```python
from build123d import *

# Parameters (mm, degrees)
SKETCH1_W                       = 0.5
SKETCH1_H                       = 16
SKETCH1_H_2                     = 1
SKETCH1_H_3                     = 3
BOSS_EXTRUDE1_DEPTH             = 15
SKETCH5_W                       = 2
SKETCH5_H                       = 3
CUT_EXTRUDE1_DEPTH              = 2
BOSS_EXTRUDE2_DEPTH             = 2
STICK_START                     = -2.8
STICK_OUTS_DEPTH                = 0.8
PIN_HOLE_SKETCH_R               = 2
PIN_HOLE_DEPTH                  = 5.183346
PIN_HOLE_DIRECTION_2_REACH      = 29.406
PIN_HOLE_DIRECTION_2_END_RADIUS = 11


with BuildPart() as part:
    # Sketch1 → Boss-Extrude1 (new body)
    with BuildSketch(Plane.XY):
        with BuildLine():
            Line((-2, -5.183346174), (-2, 10.816653826))
            ThreePointArc((-2, 10.816653826), (-7.03562364, -8.455767263), (11, 0))
            ThreePointArc((11, 0), (8.455767263, 7.03562364), (2, 10.816653826))
            Line((2, 10.816653826), (2, -5.183346174))
            Line((2, -5.183346174), (2, -6.183346174))
            Line((2, -6.183346174), (2, -9.183346174))
            Line((2, -9.183346174), (1.5, -9.183346174))
            Line((1.5, -9.183346174), (-1.5, -9.183346174))
            Line((-1.5, -9.183346174), (-2, -9.183346174))
            Line((-2, -9.183346174), (-2, -6.183346174))
            Line((-2, -6.183346174), (-1.5, -6.183346174))
            Line((-1.5, -6.183346174), (-1, -6.183346174))
            Line((-1, -6.183346174), (-1, -5.183346174))
            Line((-1, -5.183346174), (-1.5, -5.183346174))
            Line((-1.5, -5.183346174), (-2, -5.183346174))
        make_face()
        with Locations((1.75, 2.816653826)):
            Rectangle(SKETCH1_W, SKETCH1_H)
        with Locations((1.75, -5.683346174)):
            Rectangle(SKETCH1_W, SKETCH1_H_2)
        with Locations((1.75, -7.683346174)):
            Rectangle(SKETCH1_W, SKETCH1_H_3)
        with Locations((-1.75, -7.683346174)):
            Rectangle(SKETCH1_W, SKETCH1_H_3)
        with Locations((-1.75, 2.816653826)):
            Rectangle(SKETCH1_W, SKETCH1_H)
        with BuildLine():
            ThreePointArc((2, 10.816653826), (1.75046389, 10.859828552), (1.5, 10.897247359))
            Line((1.5, 10.897247359), (1.5, 10.816653826))
            Line((1.5, 10.816653826), (2, 10.816653826))
        make_face()
        with BuildLine():
            Line((-1.5, 10.816653826), (-1.5, 10.897247359))
            ThreePointArc((-1.5, 10.897247359), (-1.75046389, 10.859828552), (-2, 10.816653826))
            Line((-2, 10.816653826), (-1.5, 10.816653826))
        make_face()
    extrude(amount=BOSS_EXTRUDE1_DEPTH)

    # Sketch5 → Cut-Extrude1 (cut)
    with BuildSketch(Plane(origin=(0, 0, 0), x_dir=(-1, 0, 0), z_dir=(0, 0, -1))):
        with Locations((-5, 0)):
            Rectangle(SKETCH5_W, SKETCH5_H)
        with Locations((5, 0)):
            Rectangle(SKETCH5_W, SKETCH5_H)
    extrude(amount=-CUT_EXTRUDE1_DEPTH, mode=Mode.SUBTRACT)

    # Sketch3 → Boss-Extrude2 (add)
    with BuildSketch(Plane.XY.offset(15)):
        with BuildLine():
            add(Edge.make_bspline(
                [(-14.354093493, -5), (-12.863344749, -9.279669369), (-8.266658173, -12.812493902), (-2.2, -12.812493902)],
                knots=[0, 0, 0, 0, 1, 1, 1, 1], degree=3))
            ThreePointArc((-2.2, -12.812493902), (-8.103626672, -10.165197232), (-12, -5))
            Line((-12, -5), (-14.354093493, -5))
        make_face()
        with BuildLine():
            Line((-2.2, -12.812493902), (2.2, -12.812493902))
            ThreePointArc((2.2, -12.812493902), (8.103626672, -10.165197232), (12, -5))
            Line((12, -5), (9.797958971, -5))
            ThreePointArc((9.797958971, -5), (0, -11), (-9.797958971, -5))
            Line((-9.797958971, -5), (-12, -5))
            ThreePointArc((-12, -5), (-8.103626672, -10.165197232), (-2.2, -12.812493902))
        make_face()
        with BuildLine():
            ThreePointArc((12, -5), (8.103626672, -10.165197232), (2.2, -12.812493902))
            add(Edge.make_bspline(
                [(2.2, -12.812493902), (6.731876181, -12.812493902), (12.505086924, -10.308162631), (14.354093493, -5)],
                knots=[0, 0, 0, 0, 1, 1, 1, 1], degree=3))
            Line((14.354093493, -5), (12, -5))
        make_face()
        with BuildLine():
            ThreePointArc((-9.797958971, -5), (0, -11), (9.797958971, -5))
            Line((9.797958971, -5), (1.5, -5))
            Line((1.5, -5), (1.5, -9.183346174))
            Line((1.5, -9.183346174), (-1.5, -9.183346174))
            Line((-1.5, -9.183346174), (-1.5, -6.183346174))
            Line((-1.5, -6.183346174), (-1, -6.183346174))
            Line((-1, -6.183346174), (-1, -5.183346174))
            Line((-1, -5.183346174), (-1.5, -5.183346174))
            Line((-1.5, -5.183346174), (-1.5, -5))
            Line((-1.5, -5), (-9.797958971, -5))
        make_face()
        with BuildLine():
            Line((1.5, -5), (9.797958971, -5))
            ThreePointArc((9.797958971, -5), (10.695268783, -2.571230378), (11, 0))
            ThreePointArc((11, 0), (8.291561976, 7.228416147), (1.5, 10.897247359))
            Line((1.5, 10.897247359), (1.5, -5))
        make_face()
        with BuildLine():
            ThreePointArc((-1.5, 10.897247359), (-9.751491559, 5.090030685), (-9.797958971, -5))
            Line((-9.797958971, -5), (-1.5, -5))
            Line((-1.5, -5), (-1.5, 10.897247359))
        make_face()
        with BuildLine():
            Line((9.797958971, -5), (12, -5))
            ThreePointArc((12, -5), (12.747548784, -2.549509757), (13, 0))
            ThreePointArc((13, 0), (-2.549509757, 12.747548784), (-12, -5))
            Line((-12, -5), (-9.797958971, -5))
            ThreePointArc((-9.797958971, -5), (-9.751491559, 5.090030685), (-1.5, 10.897247359))
            ThreePointArc((-1.5, 10.897247359), (0, 11), (1.5, 10.897247359))
            ThreePointArc((1.5, 10.897247359), (8.291561976, 7.228416147), (11, 0))
            ThreePointArc((11, 0), (10.695268783, -2.571230378), (9.797958971, -5))
        make_face()
        with BuildLine():
            ThreePointArc((13, 0), (12.747548784, -2.549509757), (12, -5))
            Line((12, -5), (14.354093493, -5))
            ThreePointArc((14.354093493, -5), (14.987031412, -2.535525479), (15.2, 0))
            ThreePointArc((15.2, 0), (-2.535525479, 14.987031412), (-14.354093493, -5))
            Line((-14.354093493, -5), (-12, -5))
            ThreePointArc((-12, -5), (-2.549509757, 12.747548784), (13, 0))
        make_face()
        with BuildLine():
            ThreePointArc((1.5, 10.897247359), (0, 11), (-1.5, 10.897247359))
            Line((-1.5, 10.897247359), (1.5, 10.897247359))
        make_face()
    extrude(amount=BOSS_EXTRUDE2_DEPTH)

    # Sketch6 → Stick Outs (add)
    with BuildSketch(Plane.XY.offset(17).offset(STICK_START)):
        with BuildLine():
            Line((-11.719212261, -2.066413314), (-10.832885283, -1.910129954))
            ThreePointArc((-10.832885283, -1.910129954), (-10.973204553, -0.767321211), (-10.993299097, 0.383894464))
            Line((-10.993299097, 0.383894464), (-11.892750842, 0.415304011))
            ThreePointArc((-11.892750842, 0.415304011), (-11.871012198, -0.830102038), (-11.719212261, -2.066413314))
        make_face()
    stick_outs = extrude(amount=STICK_OUTS_DEPTH)

    # Mirror1: Stick Outs across plane
    add(stick_outs.mirror(Plane(origin=(0, 0, 0), x_dir=(0, 0, 1), z_dir=(1, 0, 0))))

    # Pin Hole sketch → Pin hole (cut)
    with BuildSketch(Plane(origin=(0, 0, 0), x_dir=(1, 0, 0), z_dir=(0, 1, 0))):
        with Locations((0, -2)):
            Circle(PIN_HOLE_SKETCH_R)
    extrude(amount=-PIN_HOLE_DEPTH, mode=Mode.SUBTRACT)

    # Pin hole direction 2: up to this cylinder (the profile starts inside it)
    pin_hole_direction_2_end = Plane(origin=(0, 0, 2), z_dir=(0, 0, -1)) * Cylinder(PIN_HOLE_DIRECTION_2_END_RADIUS, 81.812, mode=Mode.PRIVATE)
    # Pin Hole sketch → Pin hole direction 2 (cut, up to the surface)
    with BuildSketch(Plane(origin=(0, 0, 0), x_dir=(1, 0, 0), z_dir=(0, 1, 0)), mode=Mode.PRIVATE) as pin_hole_direction_2_sk1:
        with Locations((0, -2)):
            Circle(PIN_HOLE_SKETCH_R)
    pin_hole_direction_2_tool1 = extrude(pin_hole_direction_2_sk1.sketch, amount=PIN_HOLE_DIRECTION_2_REACH, mode=Mode.PRIVATE) & pin_hole_direction_2_end
    add(pin_hole_direction_2_tool1.solids().sort_by_distance((0, 0, 2))[0], mode=Mode.SUBTRACT)


solid = part.part
```
Read the model definition and answer for the solid it produces. Units are mm, in the model's axes. A direction names the side the tool comes from. Round coordinates to 2 decimals unless told otherwise and drop trailing zeros. Write each loop counter-clockwise with the first axis right and the second up, starting at its lowest first coordinate (ties: lowest second). Pieces come first, ordered by that corner, then holes. Notation, with made-up numbers: (17, 87.5) -> (73, 87.5) arc R28 cw to (73, 113.5) -> close; hole circle Ø5 at (-9.5, -21). An arc over 180 degrees is marked (long way). Answer in a Markdown table with one row per item. Add a question column.
1) Find section D-D, the plane z = 1.5. Determine the outline of the cut face in (x, y).
2) Consider line 1 (X direction, y = 4.5, z = 4.75); line 2 (X direction, y = 5.75, z = 8.75); line 3 (Z direction, x = 12, y = -2.75). Determine where each line is inside the solid, lowest interval first.
3) Find section B-B, the plane y = 10. Determine the outline of the cut face in (x, z), and give its area (3 significant figures).
4) Find section A-A, the plane x = 0. Determine the outline of the cut face in (y, z), and give its area (3 significant figures).
5) Find section C-C, the plane z = 11. Determine the outline of the cut face in (x, y).
6) Given P1, Ø0.6, axis at x = -5.5, y = 0.5, coming from the -Z side; P2, Ø1.6, axis at x = -4.5, z = 0.5, coming from the -Y side; P3, Ø5, axis at x = 11, z = 9, coming from the +Y side, each flat-ended and moving along its own axis, determine where each tip first touches the part or whether it passes through.
7) Which of the six approach directions +Z, -Z, +X, -X, +Y, -Y give full straight-line access (tool end or side, diameter ignored) to faces 5 (the face through (11.28, -1.99, 14.59)), 6 (the face through (0, 10.897, 16)), 7 (the face through (5, 0, 2))?
8) Determine the mould class of faces 1 (the face through (4, 0, 1)), 2 (the face through (0, -12.812, 16)), 3 (the face through (11.872, -0.813, 14.594)), 4 (the face through (2, 3, 2)) for opening direction X: pulls with the +X half, pulls with the -X half, needs draft (parallel to the pull), parting line crosses it, or undercut.
Findings below:
| question | item | result |
|---|---|---|
| 1 | outline | (-2, 10.82) arc R11 ccw (long way) to (2, 10.82) arc R11 ccw to (1.94, 10.83) -> (1.94, -5.18) -> (1.5, -5.18) -> (1.5, -9.18) -> (-1.5, -9.18) -> (-1.5, -6.18) -> (-1, -6.18) -> (-1, -5.18) -> (-1.94, -5.18) -> (-1.94, 10.83) arc R11 ccw to start; hole (-6, -1.5) -> (-4, -1.5) -> (-4, 1.5) -> (-6, 1.5) -> close; hole (4, -1.5) -> (6, -1.5) -> (6, 1.5) -> (4, 1.5) -> close |
| 2 | line 1 | -10.04 to -1.5, 1.5 to 10.04 |
| 2 | line 2 | -9.38 to -1.5, 1.5 to 9.38 |
| 2 | line 3 | 15 to 17 |
| 3 | outline | (-11.45, 15) -> (-4.58, 15) -> (-4.58, 0) -> (-1.5, 0) -> (-1.5, 0.68) arc R2 cw to (-1.5, 3.32) -> (-1.5, 17) -> (-11.45, 17) -> close; (1.5, 0) -> (4.58, 0) -> (4.58, 15) -> (11.45, 15) -> (11.45, 17) -> (1.5, 17) -> (1.5, 3.32) arc R2 cw to (1.5, 0.68) -> close |
| 3 | area | 130 mm² |
| 4 | outline | (-12.81, 15) -> (-11, 15) -> (-11, 0) -> (-9.18, 0) -> (-9.18, 17) -> (-12.81, 17) -> close; (10.9, 15) -> (15.2, 15) -> (15.2, 17) -> (10.9, 17) -> close |
| 4 | area | 43.1 mm² |
| 5 | outline | (-2, 10.82) arc R11 ccw (long way) to (2, 10.82) arc R11 ccw to (1.5, 10.9) -> (1.5, -9.18) -> (-1.5, -9.18) -> (-1.5, -6.18) -> (-1, -6.18) -> (-1, -5.18) -> (-1.5, -5.18) -> (-1.5, 10.9) arc R11 ccw to start |
| 6 | P1 | z = 2 |
| 6 | P2 | y = -10.36 |
| 6 | P3 | y = 6.98 |
| 7 | face 5 | -Z, -Y |
| 7 | face 6 | +Z, -Z |
| 7 | face 7 | -Z |
| 8 | face 1 | undercut |
| 8 | face 2 | needs draft |
| 8 | face 3 | pulls with the +X half |
| 8 | face 4 | undercut |
